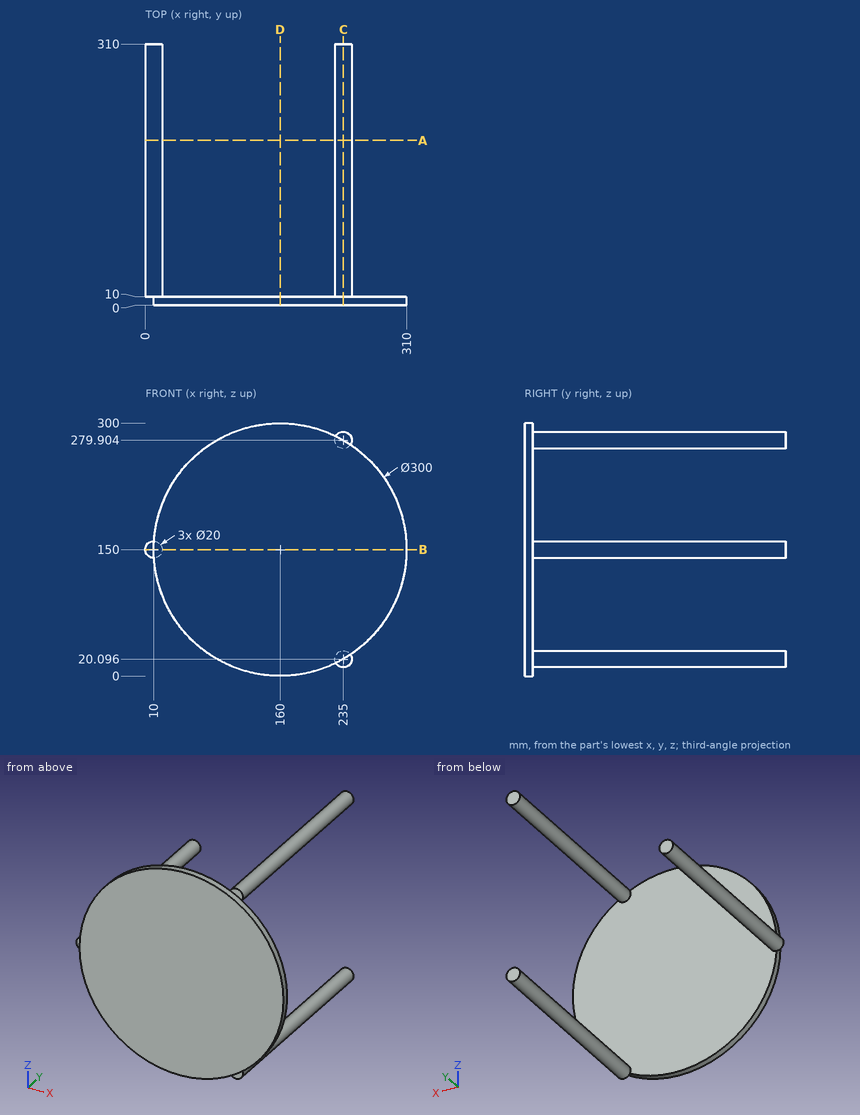
Study the drawing (mm; zero at the part's minimum x, y, z) and answer. Give positions to 0.01 mm unless a question says otherwise; leave off trailing zeros. Write each loop counter-clockwise with the first axis right and the second up, starting at its lowest first coordinate (ties: lowest second). Pieces come first, ordered by that corner, then holes. Notation, with made-up numbers: (6, 4.5) - (56, 4.5) arc R21 cw to (56, 33.5) - close; hole circle Ø1 at (29.5, 22). An arc over 180 degrees is marked (long way). Use CSV: the item, a comma, the result in double quotes. Start each with the question number.
(1) Find section A-A (y = 195.5). Give the vertices of the cut face in (x, z).
(2) Find section D-D (x = 160). Give the vertices of the cut face in (y, z), plus the area to 3 significant figures.
(3) Consider line 1 along Y through (x, z) = (55.5, 164); line 2 along X through (y, z) = (29, 276); line 3 along X through (y, z) = (76.5, 22). Determine where each line is inside the solid, lowest interval first.
(4) Find section B-B (z = 150). Give the vertices of the cut face in (x, y), plus the area to 3 significant figures.
(5) Find section C-C (x = 235). Give the vertices of the cut face in (y, z), plus the area to 3 significant figures.
(6) Given P1, Ø3, axis at x = 5, z = 146.5, coming from the -Y side; P2, Ø17, axis at x = 236, z = 18, coming from the -Y side; P3, Ø10, axis at x = 228, y = 261, coming from the -Z side; P4, Ø5, axis at x = 81, z = 132, coming from the +Y side, each flat-ended and moving along its own axis, determine where each tip first touches the part or whether it passes through.
Findings below:
1,outline,"circle Ø20 at (10, 150); circle Ø20 at (235, 20.1); circle Ø20 at (235, 279.9)"
2,outline,"(0, 0) - (10, 0) - (10, 300) - (0, 300) - close"
2,area,"3,000 mm2"
3,line 1,"0 to 10"
3,line 2,"225.79 to 244.21"
3,line 3,"225.18 to 244.82"
4,outline,"(0, 10) - (10, 10) - (10, 0) - (310, 0) - (310, 10) - (20, 10) - (20, 310) - (0, 310) - close"
4,area,"9,000 mm2"
5,outline,"(0, 20.1) - (10, 20.1) - (10, 10.1) - (310, 10.1) - (310, 30.1) - (10, 30.1) - (10, 269.9) - (310, 269.9) - (310, 289.9) - (10, 289.9) - (10, 279.9) - (0, 279.9) - close"
5,area,"14,600 mm2"
6,P1,"y = 10"
6,P2,"y = 0"
6,P3,"z = 10.3"
6,P4,"y = 10"
